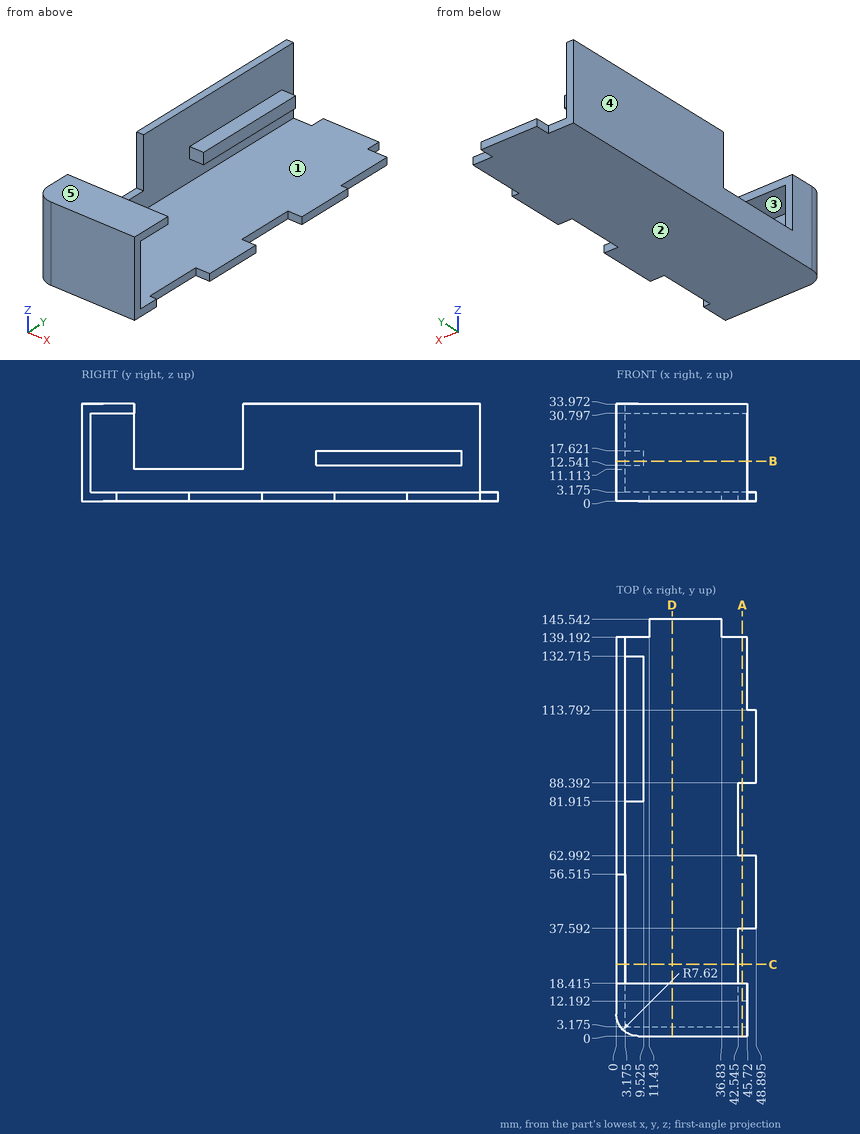
Verification items for this drawing (mm, ordinates from the low corner). A direction names the side the tool comes from. Round coordinates to 2 decimals unless told otherwise and drop trailing zeros. Write each loop counter-clockwise with the first axis right and the second up, starting at its lowest first coordinate (ties: lowest second). Pieces come first, ordered by that corner, then holes. Notation, with made-up numbers: M 12,-7 L 42,-7 A21 ccw 42,11 Z; hole C 57,6.25 d11. An arc over 180 degrees is marked long. Write item = value, one per line. Start each with the question number.
1. Section check C-C, the plane y = 25. Record the cut outline in (x, z) (1 decimal).
2. Release check for a two-part mould opening along Z. For the marked faces 3, 4 and 5 record: pulls with the +Z half, pulls with the -Z half, needs draft (parallel to the pull), parting line crosses it, or undercut.
3. Section check D-D, the plane x = 19.5. Record the cut outline in (y, z) (1 decimal).
4. Section check A-A, the plane x = 44. Record the cut outline in (y, z) (1 decimal).
5. Tool access check on the marked faces 1 and 2. Record the directions out of +Z, -Z, +X, -X, +Y, -Y that give a thin tool (end or side, any length) a straight path to the whole face; none if there is none.
6. Section check B-B, the plane z = 14. Record the cut outline in (x, y) (1 decimal), then the cut area to 3 significant figures.
7. Gauge pin test, flat ends, axial feed: pin 1 (7 mm diameter, centred on x = 7, y = 117, fed in from +Z); pin 2 (4 mm diameter, centred on x = 37.5, y = 116.5, fed in from +Z) (1 decimal); pin 3 (5.5 mm diameter, centred on x = 6.5, z = 14.5, fed in from +Y) (1 decimal). Record the tip position at first contact, or that the pin passes through.
8. Scan lines: line 1 (Z direction, x = 38.5, y = 13.5) (1 decimal); line 2 (Z direction, x = 29.5, y = 135.5) (1 decimal). Record each from-to range of solid material in increasing order. Write a range as [from, to].
Results found:
q1.outline = M 0,0 L 42.5,0 L 42.5,3.2 L 3.2,3.2 L 3.2,11.1 L 0,11.1 Z
q2.face_3 = undercut
q2.face_4 = needs draft
q2.face_5 = pulls with the +Z half
q3.outline = M 0,0 L 145.5,0 L 145.5,3.2 L 3.2,3.2 L 3.2,30.8 L 18.4,30.8 L 18.4,34 L 0,34 Z
q4.outline = M 0,0 L 12.2,0 L 12.2,3.2 L 3.2,3.2 L 3.2,30.8 L 18.4,30.8 L 18.4,34 L 0,34 Z; M 37.6,0 L 63,0 L 63,3.2 L 37.6,3.2 Z; M 88.4,0 L 139.2,0 L 139.2,3.2 L 88.4,3.2 Z
q5.face_1 = +X, +Y
q5.face_2 = -Z, +X, -X, +Y, -Y
q6.outline = M 0,7.6 A7.6 ccw 7.6,0 L 45.7,0 L 45.7,3.2 L 3.2,3.2 L 3.2,18.4 L 0,18.4 Z; M 0,56.5 L 3.2,56.5 L 3.2,81.9 L 9.5,81.9 L 9.5,132.7 L 3.2,132.7 L 3.2,139.2 L 0,139.2 Z
q6.area = 766 mm^2
q7.pin_1 = 17.62
q7.pin_2 = 3.2
q7.pin_3 = 132.7
q8.line_1 = [0, 3.2], [30.8, 34]
q8.line_2 = [0, 3.2]
